For this review, use the dimensioned drawing (mm, ordinates from the lowest corner) and the shaded views. A direction names the side the tool comes from. Round coordinates to 2 decimals unless told otherwise and drop trailing zeros. Write each loop counter-clockwise with the first axis right and the second up, starting at its lowest first coordinate (ties: lowest second). Pieces come first, ordered by that corner, then holes. Notation, with made-up numbers: (51, -0.5) - (66, -0.5) arc R32 ccw to (66, 31.5) - close; hole circle Ø9 at (50, 81.5). An arc over 180 degrees is marked (long way). Write each question's results on one line, items separated by ' | '.
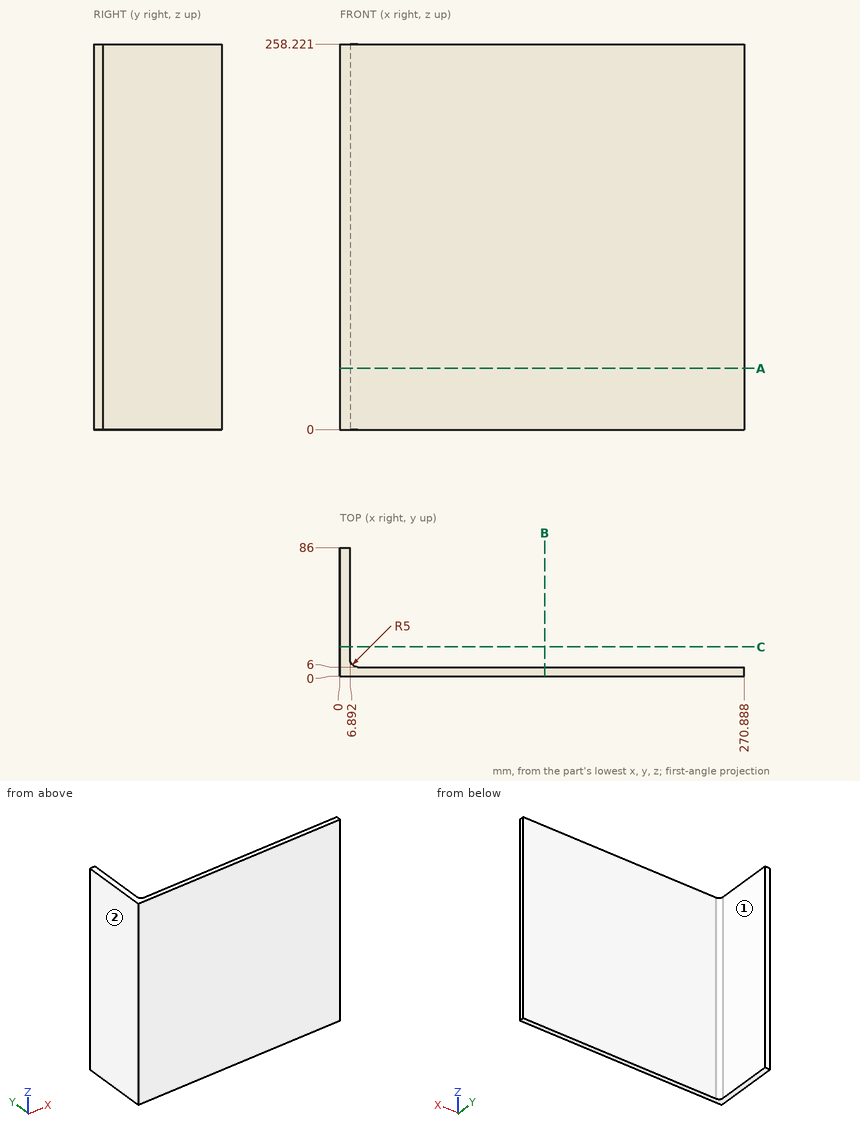
Q1. We need section B-B (x = 137). State the section outline as (y, z) points, plus the area to 3 significant figures.
Evaluation:
outline: (0, 0) - (6, 0) - (6, 258.22) - (0, 258.22) - close | area: 1,550 mm^2
Q2. Tool access review of the marked faces 1 and 2: name each direction out of +Z, -Z, +X, -X, +Y, -Y from which nothing blocks a thin tool from reaching the whole face with its end or side.
Evaluation:
face 1: +Z, -Z, +X, +Y | face 2: +Z, -Z, -X, +Y, -Y
Q3. We need section C-C (y = 19.5). State the section outline as (x, z) points.
Evaluation:
outline: (0, 0) - (6.89, 0) - (6.89, 258.22) - (0, 258.22) - close
Q4. Insertion check: P1, Ø2, axis at x = 69.5, z = 145.5, coming from the +Y side; P2, Ø8, axis at y = 58.5, z = 160.5, coming from the +X side. Each pin has a flat end and moves straight along its axis. Give the tip position at first contact, or say it passes through.
Evaluation:
P1: stops at y = 6 | P2: stops at x = 6.89
Q5. We need section A-A (z = 41). State the section outline as (x, y) points.
Evaluation:
outline: (0, 0) - (270.89, 0) - (270.89, 6) - (11.89, 6) arc R5 cw to (6.89, 11) - (6.89, 86) - (0, 86) - close
Q6. For probe 1 along X at (y, z) = (16.5, 16.5); probe 2 along Y at (x, z) = (192, 166.5), list the stretches that pass through material, from the lowest coordinate up.
Evaluation:
probe 1: x = 0 to 6.89 | probe 2: y = 0 to 6
